Build history of the part. All positions in model axes, mm. Give positions to 0.01 mm unless a question says otherwise; leave off trailing zeros. Answer as a JSON object with one key per item and string values. Group by question number.
Q1. Two-plate mould, pull along X, no slides. Class faces 1 (the cylindrical face through (23.02, 13.13, 0.23)), 2 (the flat face through (-7, 0, -16.5)), 3 (the cylindrical face through (-1.518, -6.221, -0.231)): pulls with the +X half, pulls with the -X half, needs draft (parallel to the pull), parting line crosses it, or undercut.
Q2. Drop flat-ended pins along their axis: pin 1 (19 mm diameter, centred on x = -14, z = 2.5, fed in from +Y); pin 2 (8 mm diameter, centred on x = 15.5, z = -6.5, fed in from +Y); pin 3 (1 mm diameter, centred on y = -2.5, z = -12, fed in from -X); pin 4 (10 mm diameter, centred on x = -1.5, z = 0, fed in from -Y). Give the stop position or say it passes through.
Q3. Wall check: probe 1 along Y at (x, z) = (19.5, 6.5); probe 2 along Y at (x, z) = (-5, 7); probe 3 along Y at (x, z) = (0, -1). Give the ranges that are in metal, low to high. Write a range as from..to.
Q4. Band-saw the part on A-A, the plane z = 13. Count the separate pieces of the cut face and the enclosed holes in it, plus the area to 3 significant figures.
from build123d import *

# Parameters (mm, degrees)
SCHNITT_LINEAR_AUSTRAGEN1_DEPTH = 34.0000001
VERRUNDUNG1_R                   = 2
KREISMUSTER1_COUNT              = 6
VERRUNDUNG1_OF_KREISMUSTER1_R   = 2
SKIZZE7_R                       = 2.5
SCHNITT_LINEAR_AUSTRAGEN3_DEPTH = 34.0000001


with BuildPart() as part:
    # Skizze4 → Rotation1 (revolve)
    with BuildSketch(Plane(origin=(0, 0, 0), x_dir=(0, 0, -1), z_dir=(1, 0, 0))):
        with BuildLine():
            Line((-16.5, 31.5), (-16.5, 0))
            Line((-16.5, 0), (16.5, 0))
            Line((16.5, 0), (16.5, 31.5))
            ThreePointArc((16.5, 31.5), (0, 34), (-16.5, 31.5))
        make_face()
    revolve(axis=Axis((0, 0, 6.739526199), (0, 0, -1)))

    # Skizze5 → Schnitt-Linear austragen1 (cut, through all)
    with BuildSketch(Plane.XY.offset(16.5)):
        with BuildLine():
            Line((-11.92971845, 23.662878475), (-1.605699404, 5.781152949))
            ThreePointArc((-1.605699404, 5.781152949), (0, 6), (1.605699404, 5.781152949))
            Line((1.605699404, 5.781152949), (11.92971845, 23.662878475))
            ThreePointArc((11.92971845, 23.662878475), (0, 26.5), (-11.92971845, 23.662878475))
        make_face()
    schnitt_linear_austragen1 = extrude(amount=-SCHNITT_LINEAR_AUSTRAGEN1_DEPTH, mode=Mode.SUBTRACT)

    # Verrundung1
    verrundung1_edges = [part.edges().sort_by_distance(p)[0] for p in [
        (-11.92971845, 23.662878475, 0),
        (11.92971845, 23.662878475, 0),
        (1.605699404, 5.781152949, 0),
        (-1.605699404, 5.781152949, 0),
    ]]
    fillet(verrundung1_edges, radius=VERRUNDUNG1_R)

    # Kreismuster1: Schnitt-Linear austragen1 ×6 about axis
    kreismuster1_axis = Axis((0, 0, 0), (0, 0, 1))
    for i in range(1, KREISMUSTER1_COUNT):
        add(schnitt_linear_austragen1.rotate(kreismuster1_axis, i * 360 / KREISMUSTER1_COUNT), mode=Mode.SUBTRACT)

    # Verrundung1 of Kreismuster1
    verrundung1_of_kreismuster1_edges = [part.edges().sort_by_distance(p)[0] for p in [
        (-26.457513111, 1.5, 0),
        (-14.527794661, 22.162878475, 0),
        (-4.203775615, 4.281152949, 0),
        (-5.809475019, 1.5, 0),
        (-14.527794661, -22.162878475, 0),
        (-26.457513111, -1.5, 0),
        (-5.809475019, -1.5, 0),
        (-4.203775615, -4.281152949, 0),
        (11.92971845, -23.662878475, 0),
        (-11.92971845, -23.662878475, 0),
        (-1.605699404, -5.781152949, 0),
        (1.605699404, -5.781152949, 0),
        (26.457513111, -1.5, 0),
        (14.527794661, -22.162878475, 0),
        (4.203775615, -4.281152949, 0),
        (5.809475019, -1.5, 0),
        (14.527794661, 22.162878475, 0),
        (26.457513111, 1.5, 0),
        (5.809475019, 1.5, 0),
        (4.203775615, 4.281152949, 0),
    ]]
    fillet(verrundung1_of_kreismuster1_edges, radius=VERRUNDUNG1_OF_KREISMUSTER1_R)

    # Skizze7 → Schnitt-Linear austragen3 (cut, through all)
    with BuildSketch(Plane.XY.offset(16.5)):
        Circle(SKIZZE7_R)
    extrude(amount=-SCHNITT_LINEAR_AUSTRAGEN3_DEPTH, mode=Mode.SUBTRACT)


solid = part.part
Worked answers:
{
 "1": {"face 1": "undercut", "face 2": "needs draft", "face 3": "undercut"},
 "2": {"pin 1": "y = 33.68", "pin 2": "y = 31.66", "pin 3": "x = -32.71", "pin 4": "y = -34"},
 "3": {"probe 1": "-27.39..-17.94, -1.5..1.5, 17.94..27.39", "probe 2": "-33.18..-26.02, -11.66..-5.66, -3.32..3.32, 5.66..11.66, 26.02..33.18", "probe 3": "-33.99..-26.5, -6..-2.5, 2.5..6, 26.5..33.99"},
 "4": {"separate pieces": "1", "enclosed holes": "7", "area": "1,580 mm2"}
}
